from build123d import *

# Parameters (mm, degrees)
SKETCH1_R           = 2.55
BOSS_EXTRUDE1_DEPTH = 52
BOSS_EXTRUDE2_DEPTH = 8
CUT_EXTRUDE1_DEPTH  = 1.525
SKETCH4_R           = 2.55
CUT_EXTRUDE2_DEPTH  = 62.43329716


with BuildPart() as part:
    # Sketch1 → Boss-Extrude1 (new body)
    with BuildSketch(Plane(origin=(0, 0, 0), x_dir=(1, 0, 0), z_dir=(0, 1, 0))):
        with BuildLine():
            Line((-3, -5.9), (3, -5.9))
            ThreePointArc((3, -5.9), (5.050609665, -5.050609665), (5.9, -3))
            Line((5.9, -3), (5.9, 3))
            ThreePointArc((5.9, 3), (5.050609665, 5.050609665), (3, 5.9))
            Line((3, 5.9), (-3, 5.9))
            ThreePointArc((-3, 5.9), (-5.050609665, 5.050609665), (-5.9, 3))
            Line((-5.9, 3), (-5.9, -3))
            ThreePointArc((-5.9, -3), (-5.050609665, -5.050609665), (-3, -5.9))
        make_face()
        with Locations(Location((0, 0, 0), (0, 0, 90))):
            Circle(SKETCH1_R, mode=Mode.SUBTRACT)
    extrude(amount=BOSS_EXTRUDE1_DEPTH)

    # Sketch2 → Boss-Extrude2 (add)
    with BuildSketch(Plane(origin=(0, 52, 0), x_dir=(1, 0, 0), z_dir=(0, 1, 0))):
        with BuildLine():
            Line((5.9, -3), (5.9, 3))
            ThreePointArc((5.9, 3), (5.050609665, 5.050609665), (3, 5.9))
            Line((3, 5.9), (-3, 5.9))
            ThreePointArc((-3, 5.9), (-5.050609665, 5.050609665), (-5.9, 3))
            Line((-5.9, 3), (-5.9, -3))
            ThreePointArc((-5.9, -3), (-5.050609665, -5.050609665), (-3, -5.9))
            Line((-3, -5.9), (3, -5.9))
            ThreePointArc((3, -5.9), (5.050609665, -5.050609665), (5.9, -3))
        make_face()
    extrude(amount=BOSS_EXTRUDE2_DEPTH)

    # Sketch3 → Cut-Extrude1 (cut, symmetric)
    with BuildSketch(Plane(origin=(0, 3, 0), x_dir=(-1, 0, 0), z_dir=(0, -1, 0))):
        Polygon((2.742413779, 4.75), (6.305323331, 4.75), (6.305323331, -4.75), (2.742413779, -4.75), (-2.742413779, -4.75), (-5.484827557, 0), (-2.742413779, 4.75), align=None)
    extrude(amount=CUT_EXTRUDE1_DEPTH, both=True, mode=Mode.SUBTRACT)

    # Sketch4 → Cut-Extrude2 (cut, through all)
    with BuildSketch(Plane(origin=(0, 0, -5.9), x_dir=(-1, 0, 0), z_dir=(0, 0, -1))):
        with Locations((0, 55.5)):
            Circle(SKETCH4_R)
    extrude(amount=-CUT_EXTRUDE2_DEPTH, mode=Mode.SUBTRACT)


solid = part.part
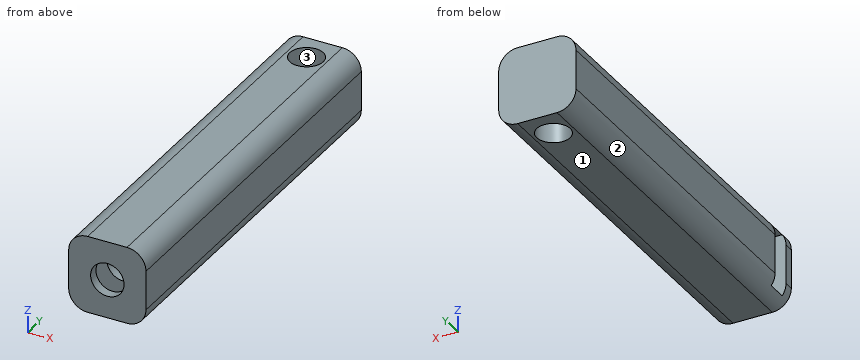
Source: CAD feature listing. Evaluate the final solid. Frame: model axes, mm. Face numbers are marked on the shaded views. Round coordinates to 2 decimals unless told otherwise and drop trailing zeros. Loops run counter-clockwise (first coordinate to the right, second up) from the corner with the lowest first, then second, coordinate; pieces in that order, holes last. Notation, with made-up numbers: M 25.25,-31 L 31.25,-31 A25 cw 31.25,-11 Z; hole C 0,38 d2. An arc over 180 degrees is marked long. Return JSON: item names as keys, results as strings. Group by question number.
1. Material intervals for line 1 along X through (y, z) = (31.5, 0); line 2 along Y through (x, z) = (-1.5, -3.25) (3 decimals); line 3 along Y through (x, z) = (-4.5, 3) (3 decimals), sorted ascending. Write a range as from..to.
2. Pin query (flat end, axial travel): pin 1 (4 mm diameter, centred on x = 0, y = 55.5, fed in from -Z); pin 2 (2.5 mm diameter, centred on x = 0.5, z = -0.5, fed in from -Y). Return the tip coordinate at first contact, or that it passes through.
3. Mould query, pull axis X, two halves, no side actions, for the marked faces 1, 2 and 3. Classes: released by +X, released by -X, zero draft, split by the parting line, or undercut.
4. Section query C-C on y = 55.5. Output: boundary loops of the cut face in (x, z).
5. Section query B-B on x = 0. Output: boundary loops of the cut face in (y, z) (3 decimals).
6. Section query D-D on z = 1.75. Output: boundary loops of the cut face in (x, y) (3 decimals), and give its area (3 significant figures).
7. Section query A-A on y = 26. Output: boundary loops of the cut face in (x, z).
Checks:
{
 "1": {"line 1": "x = -5.9..-2.55, 2.55..5.9", "line 2": "y = 0..1.475, 4.525..53.438, 57.562..60", "line 3": "y = 0..1.475, 4.525..60"},
 "2": {"pin 1": "passes through", "pin 2": "stops at y = 52"},
 "3": {"face 1": "zero draft", "face 2": "released by -X", "face 3": "undercut"},
 "4": {"outline": "M -5.9,-3 A2.9 ccw -3,-5.9 L -2.55,-5.9 L -2.55,5.9 L -3,5.9 A2.9 ccw -5.9,3 Z; M 2.55,-5.9 L 3,-5.9 A2.9 ccw 5.9,-3 L 5.9,3 A2.9 ccw 3,5.9 L 2.55,5.9 Z"},
 "5": {"outline": "M 0,-5.9 L 52.95,-5.9 L 52.95,5.9 L 0,5.9 L 0,2.55 L 1.475,2.55 L 1.475,4.75 L 4.525,4.75 L 4.525,2.55 L 52,2.55 L 52,-2.55 L 4.525,-2.55 L 4.525,-4.75 L 1.475,-4.75 L 1.475,-2.55 L 0,-2.55 Z; M 58.05,-5.9 L 60,-5.9 L 60,5.9 L 58.05,5.9 Z"},
 "6": {"outline": "M -5.9,0 L -1.855,0 L -1.855,1.475 L -5.9,1.475 Z; M -5.9,4.525 L -1.855,4.525 L -1.855,52 L 1.855,52 L 1.855,4.525 L 4.474,4.525 L 4.474,1.475 L 1.855,1.475 L 1.855,0 L 5.9,0 L 5.9,60 L -5.9,60 Z; hole C 0,55.5 d5.1", "area": "474 mm²"},
 "7": {"outline": "M -5.9,-3 A2.9 ccw -3,-5.9 L 3,-5.9 A2.9 ccw 5.9,-3 L 5.9,3 A2.9 ccw 3,5.9 L -3,5.9 A2.9 ccw -5.9,3 Z; hole C 0,0 d5.1"}
}
